Part model, mm, in its own coordinate system. Face numbers are marked on the shaded views. Coordinates: 2 decimals unless noted, no trailing zeros. Loops run counter-clockwise (first coordinate to the right, second up) from the corner with the lowest first, then second, coordinate; pieces in that order, holes last. Notation, with made-up numbers: (-38, -8) - (7, -8) arc R9 ccw to (7, 9) - close; hole circle Ø8 at (78.5, 26.5). An arc over 180 degrees is marked (long way). Use a Markdown table: item, result. Add a question column.
1) Probe probe 1 along X at (y, z) = (1, 1.7); probe 2 along Y at (x, z) = (-6.5, 2); probe 3 along Y at (x, z) = (12.5, 0.95). List the from-to ranges inside material, lowest first. Write a range as [from, to].
2) Band-saw the part on B-B (y = -13). Give the cut face in (x, z).
3) Drop flat-ended pins along their axis: P1, Ø2, axis at x = 0, y = 12.5, coming from the -Z side (1 decimal); P2, Ø1.5, axis at x = -13.5, z = 0.5, coming from the -Y side; P3, Ø1, axis at x = 6.5, z = 2.5, coming from the -Y side; P4, Ø1.5, axis at y = 12, z = 1.5, coming from the +X side. Give the stop position or say it passes through.
4) Pull direction Y, two halves, no side cores. Call the marked faces 1, 2 and 3: +Y half, -Y half, draft (parallel to the pull), parting line (faces both ways), or undercut.
5) Band-saw the part on C-C (x = -12.5). Give the cut face in (y, z), plus the area to 3 significant figures.
6) Band-saw the part on D-D (z = 2.2). Give the number of separate pieces and of enclosed holes in the cut face, plus the area to 3 significant figures.
7) Band-saw the part on A-A (y = 0). Give the cut face in (x, z), plus the area to 3 significant figures.
Autodesk Fusion 360 part; units mm, degrees
sketch "草图1" plane through (0, 0, 0) normal (0, 0, 1) x (1, 0, 0)
  line L0 (0, 0) -> (51.8, 0) construction
  line L1 (0, 0) -> (0, 48.8683) construction
  circle A0 centre (0, 0) radius 18
  circle A1 centre (0, 0) radius 5
  line L2 (0, 0) -> (20.6611, 20.6611) construction
  line L3 (0, 0) -> (29.2192, 0) construction
  line L4 (0, 0) -> (15.4724, -15.4724) construction
  line L5 (0, 0) -> (21.8812, 0) construction
  point P0 (6.7175, 6.7175)
  point P1 (5.6569, -5.6569)
  point P2 (-6.7175, -6.7175)
  point P3 (-5.6569, 5.6569)
  point P4 (12.5, 0)
  point P5 (-12.5, 0)
  point P6 (0, -12.5)
  point P7 (0, 12.5)
  dimension "d1" = 36
  dimension "d2" = 10
  dimension "d3" = 45
  dimension "d4" = 45
  dimension "d5" = 9.5
  dimension "d6" = 8
  dimension "d7" = 12.5
extrude "拉伸1" add sketch "草图1" along normal blind 3
sketch "草图3" plane through (0, 0, 3) normal (0, 0, 1) x (-1, 0, 0)
  circle A0 centre (0, 0) radius 5
  circle A1 centre (0, 0) radius 18
  line L0 (0, 0) -> (-31, 0) construction
  line L1 (0, 0) -> (17.0073, -17.0073) construction
  line L2 (0, 0) -> (27.2176, 0) construction
  line L3 (0, 0) -> (-13.435, -13.435) construction
  point P0 (-6.7175, -6.7175)
  point P1 (5.6569, -5.6569)
  point P2 (6.7175, 6.7175)
  point P3 (-5.6569, 5.6569)
  dimension "d10" = 45
  dimension "d11" = 45
  dimension "d12" = 9.5
  dimension "d13" = 8
hole "孔1" at (6.7175, 6.7175, 3) at (-5.6569, 5.6569, 3) at (-6.7175, -6.7175, 3) at (5.6569, -5.6569, 3) direction (0, 0, -1) diameter 3 depth 5 tip angle 118 countersink diameter 6 countersink angle 90
sketch "草图4" plane through (0, 0, 3) normal (0, 0, 1) x (-1, 0, 0)
  circle A0 centre (0, 0) radius 18
  arc A1 (3.5355, -3.5355) -> (-3.5355, 3.5355) centre (0, 0) ccw
  circle A2 centre (5.6569, -5.6569) radius 3
  arc A3 (-3.5355, 3.5355) -> (3.5355, -3.5355) centre (0, 0) ccw
  circle A4 centre (-5.6569, 5.6569) radius 3
  circle A5 centre (-6.7175, -6.7175) radius 3
  circle A6 centre (6.7175, 6.7175) radius 3
  line L0 (0, 0) -> (-28, 0) construction
  line L1 (0, 0) -> (0, -25) construction
  line L2 (0, 0) -> (-17, -17) construction
  point P0 (0, -12.5)
  point P1 (0, 12.5)
  point P2 (-12.5, 0)
  point P3 (12.5, 0)
  dimension "d19" = 12.5
  dimension "d20" = 45
hole "孔2" at (0, 12.5, 3) at (-12.5, 0, 3) at (0, -12.5, 3) at (12.5, 0, 3) direction (0, 0, -1) diameter 2.529 depth 5 tip angle 118
sketch "草图5" plane through (0, 0, 0) normal (0, 0, -1) x (1, 0, 0)
  circle A0 centre (0, 12.5) radius 1.2645
  circle A1 centre (0, -12.5) radius 1.2645
  circle A2 centre (-12.5, 0) radius 1.2645
  circle A3 centre (12.5, 0) radius 1.2645
  circle A4 centre (-6.7175, 6.7175) radius 1.5
  circle A5 centre (6.7175, -6.7175) radius 1.5
  circle A6 centre (-5.6569, -5.6569) radius 1.5
  circle A7 centre (5.6569, 5.6569) radius 1.5
  circle A8 centre (0, 0) radius 5
  circle A9 centre (0, 0) radius 18
equation "d7 = ( 25 / 2 ) * 1 mm"
equation "d19 = ( 25 / 2 ) * 1 mm"
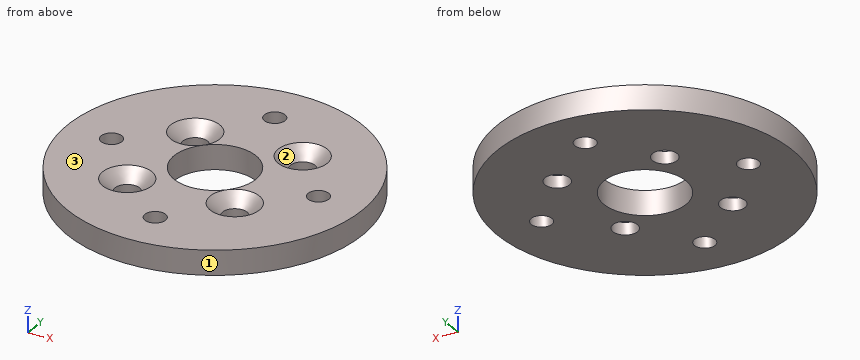
Answer block:
| question | item | result |
|---|---|---|
| 1 | probe 1 | [-17.97, -13.27], [-11.73, -4.9], [4.9, 11.73], [13.27, 17.97] |
| 1 | probe 2 | [-16.79, -8.71], [-4.73, 3.84], [7.47, 16.79] |
| 1 | probe 3 | [-12.95, -1.26], [1.26, 12.95] |
| 2 | outline | (-12.45, 0) - (-1.16, 0) - (-1.16, 3) - (-12.45, 3) - close; (1.16, 0) - (12.45, 0) - (12.45, 3) - (1.16, 3) - close |
| 3 | P1 | through |
| 3 | P2 | y = -12.71 |
| 3 | P3 | y = -16.97 |
| 3 | P4 | x = 14.05 |
| 4 | face 1 | parting line |
| 4 | face 2 | undercut |
| 4 | face 3 | draft |
| 5 | outline | (-12.95, 0) - (-1.26, 0) - (-1.26, 3) - (-12.95, 3) - close; (1.26, 0) - (12.95, 0) - (12.95, 3) - (1.26, 3) - close |
| 5 | area | 70.1 mm2 |
| 6 | separate pieces | 1 |
| 6 | enclosed holes | 9 |
| 6 | area | 858 mm2 |
| 7 | outline | (-18, 0) - (-13.76, 0) - (-13.76, 3) - (-18, 3) - close; (-11.24, 0) - (-5, 0) - (-5, 3) - (-11.24, 3) - close; (5, 0) - (11.24, 0) - (11.24, 3) - (5, 3) - close; (13.76, 0) - (18, 0) - (18, 3) - (13.76, 3) - close |
| 7 | area | 62.8 mm2 |
